Check sheet for the drawn part. Datum: minimum x, y, z corner. Units: mm. A direction names the side the tool comes from. Round coordinates to 2 decimals unless told otherwise and drop trailing zeros. Write each loop counter-clockwise with the first axis right and the second up, starting at its lowest first coordinate (ties: lowest second). Pieces come first, ordered by that corner, then holes.
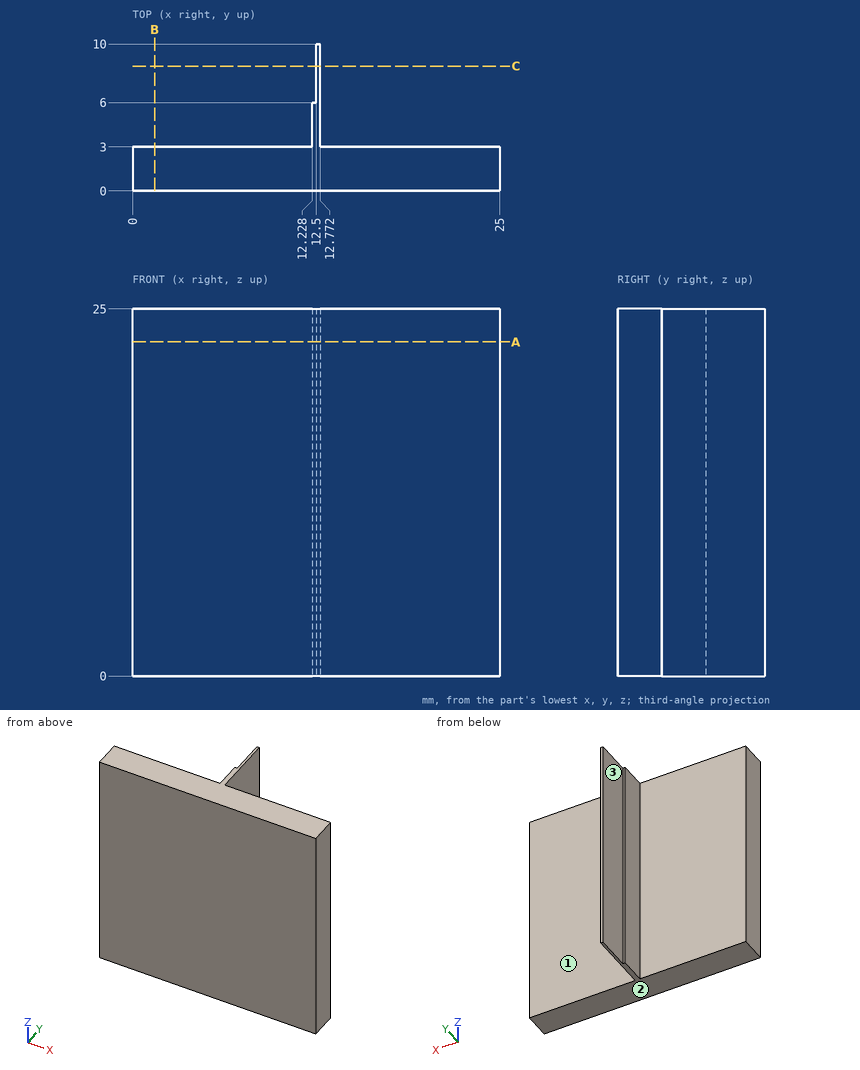
Q1. Sectioned sample at A-A (z = 22.75). Enter the section's corners in (x, y), plus the area to 3 significant figures.
Recorded:
outline: (0, 0) - (25, 0) - (25, 3) - (12.77, 3) - (12.77, 10) - (12.5, 10) - (12.5, 6) - (12.23, 6) - (12.23, 3) - (0, 3) - close
area: 77.7 mm2
Q2. Sectioned sample at B-B (x = 1.5). Enter the section's corners in (y, z).
Recorded:
outline: (0, 0) - (3, 0) - (3, 25) - (0, 25) - close
Q3. Tool access check on the marked faces 1, 2 and 3. Record the directions out of +Z, -Z, +X, -X, +Y, -Y that give a thin tool (end or side, any length) a straight path to the whole face; none if there is none.
Recorded:
face 1: +Z, -Z, +X, +Y
face 2: -Z, +X, -X, +Y, -Y
face 3: +Z, -Z, -X, +Y
Q4. Material ranges on line 1 along Y through (x, z) = (13, 15); line 2 along X through (y, z) = (8.5, 8); line 3 along X through (y, z) = (5, 4.25), recorded low to high.
Recorded:
line 1: y = 0 to 3
line 2: x = 12.5 to 12.77
line 3: x = 12.23 to 12.77
Q5. Sectioned sample at C-C (y = 8.5). Enter the section's corners in (x, z), plus the area to 3 significant figures.
Recorded:
outline: (12.5, 0) - (12.77, 0) - (12.77, 25) - (12.5, 25) - close
area: 6.80 mm2
Q6. Depth check by flat-ended pin: P1, Ø0.9, axis at y = 4.5, z = 7, coming from the -X side; P2, Ø5.5, axis at y = 6.5, z = 12.5, coming from the +X side; P3, Ø1, axis at x = 3, z = 10, coming from the +Y side. Enter the tip coordinate at first touch or a pass-through.
Recorded:
P1: stops at x = 12.23
P2: stops at x = 12.77
P3: stops at y = 3
